from build123d import *

# Parameters (mm, degrees)
BOSS_EXTRUDE1_DEPTH = 200
CUT_EXTRUDE1_START  = -2
CUT_EXTRUDE1_DEPTH  = 196
BOSS_EXTRUDE3_DEPTH = 50
SKETCH6_W           = 200
SKETCH6_H           = 50
BOSS_EXTRUDE4_DEPTH = 10


with BuildPart() as part:
    # Sketch1 → Boss-Extrude1 (new body)
    with BuildSketch(Plane.XY):
        with BuildLine():
            Line((0, 0), (0, 21.170605096))
            ThreePointArc((0, 21.170605096), (200, 54.314575051), (400, 21.170605096))
            Line((400, 21.170605096), (400, 0))
            ThreePointArc((400, 0), (200, 34.314575051), (0, 0))
        make_face()
    extrude(amount=BOSS_EXTRUDE1_DEPTH)

    # Sketch3 → Cut-Extrude1 (cut)
    with BuildSketch(Plane.XY.offset(200).offset(CUT_EXTRUDE1_START)):
        with BuildLine():
            Line((2, 1.762370006), (2, 0.703134257))
            ThreePointArc((2, 0.703134257), (200, 34.314575051), (398, 0.703134257))
            Line((398, 0.703134257), (398, 1.762370006))
            ThreePointArc((398, 1.762370006), (200, 35.314575051), (2, 1.762370006))
        make_face()
    extrude(amount=-CUT_EXTRUDE1_DEPTH, mode=Mode.SUBTRACT)

    # Sketch5 → Boss-Extrude3 (add)
    with BuildSketch(Plane(origin=(0, 0, 0), x_dir=(-1, 0, 0), z_dir=(0, 0, -1))):
        with BuildLine():
            Line((-210, 50.233400871), (-210, 38.23178792))
            ThreePointArc((-210, 38.23178792), (-200, 38.314575051), (-190, 38.23178792))
            Line((-190, 38.23178792), (-190, 50.233400871))
            ThreePointArc((-190, 50.233400871), (-200, 50.314575051), (-210, 50.233400871))
        make_face()
    extrude(amount=BOSS_EXTRUDE3_DEPTH)

    # Sketch6 → Boss-Extrude4 (add)
    with BuildSketch(Plane(origin=(0, 0, -50), x_dir=(-1, 0, 0), z_dir=(0, 0, -1))):
        with Locations((-200, 39.232594396)):
            Rectangle(SKETCH6_W, SKETCH6_H)
    extrude(amount=BOSS_EXTRUDE4_DEPTH)


solid = part.part
The listing builds one solid part. Answer for the finished solid, in the listing's coordinates (mm). A direction names the side the tool comes from. Give positions to 0.01 mm unless a question says otherwise; leave off trailing zeros. Loops run counter-clockwise (first coordinate to the right, second up) from the corner with the lowest first, then second, coordinate; pieces in that order, holes last. Notation, with made-up numbers: M -26,79.25 L -14,79.25 A22 ccw -14,116.25 Z; hole C -14.75,27.5 d9. An arc over 180 degrees is marked long. Answer as CSV lines item,"result".
Item 1: Given pin 1 Ø11 at (x, z) = (213.5, -54) entering from -Y; pin 2 Ø1.5 at (x, z) = (193.5, 93) entering from +Y; pin 3 Ø3 at (y, z) = (38, -56.5) entering from -X, each flat-ended and moving along its own axis, determine where each tip first touches the part or whether it passes through.
Values follow:
pin 1,"stops at y = 14.23"
pin 2,"stops at y = 54.29"
pin 3,"stops at x = 100"
Item 2: The part is cut by section B-B (z = 90.5). Give the vertices of the cut face in (x, y).
Values follow:
outline,"M 0,0 A600 cw 2,0.7 L 2,1.76 A601 cw 398,1.76 L 398,0.7 A600 cw 400,0 L 400,21.17 A620 ccw 0,21.17 Z"
Item 3: Which of the six approach directions +Z, -Z, +X, -X, +Y, -Y give full straight-line access (tool end or side, diameter ignored) to faces 1 (the flat face through (214, 35, 198)), 2 (the cylindrical face through (197.15, 54.31, 98.6)), 3 (the flat face through (210, 44, -25))?
Values follow:
face 1,"-Y"
face 2,"+Z, +Y"
face 3,"+X, +Y, -Y"
Item 4: The mould has two halves that part along Z. Classify faces 4 (the flat face through (201, 64.233, -55)), 5 (the flat face through (203, 40, 200)), 6 (the cylindrical face through (202.825, 35.308, 101.372)), 7 (the flat face through (214, 35, 2)): released by +Z, released by -Z, zero draft, split by the parting line, or undercut.
Values follow:
face 4,"zero draft"
face 5,"released by +Z"
face 6,"undercut"
face 7,"undercut"
Item 5: The part is cut by section A-A (x = 244.5). Give the vertices of the cut face in (y, z).
Values follow:
outline,"M 14.23,-60 L 64.23,-60 L 64.23,-50 L 14.23,-50 Z; M 32.66,0 L 52.72,0 L 52.72,200 L 32.66,200 L 32.66,198 L 33.66,198 L 33.66,2 L 32.66,2 Z"
Item 6: Straight lines are drawn through the part: line 1 along Z through (x, y) = (217, 35); line 2 along Z through (x, y) = (118, 49.5); line 3 along Z through (x, y) = (182, 48). For each, find the intervals that lie inside material, in ascending order. Write a range as [from, to].
Values follow:
line 1,"z = [-60, -50], [0, 2], [198, 200]"
line 2,"z = [-60, -50]"
line 3,"z = [-60, -50], [0, 200]"
Item 7: The part is cut by section D-D (x = 308.5). Give the vertices of the cut face in (y, z), and give its area (3 significant figures).
Values follow:
outline,"M 24.42,0 L 44.75,0 L 44.75,200 L 24.42,200 L 24.42,198 L 25.44,198 L 25.44,2 L 24.42,2 Z"
area,"3,870 mm^2"
Item 8: The part is cut by section C-C (x = 118). Give the vertices of the cut face in (y, z), and give its area (3 significant figures).
Values follow:
outline,"M 14.23,-60 L 64.23,-60 L 64.23,-50 L 14.23,-50 Z; M 28.68,0 L 48.87,0 L 48.87,200 L 28.68,200 L 28.68,198 L 29.69,198 L 29.69,2 L 28.68,2 Z"
area,"4,340 mm^2"
